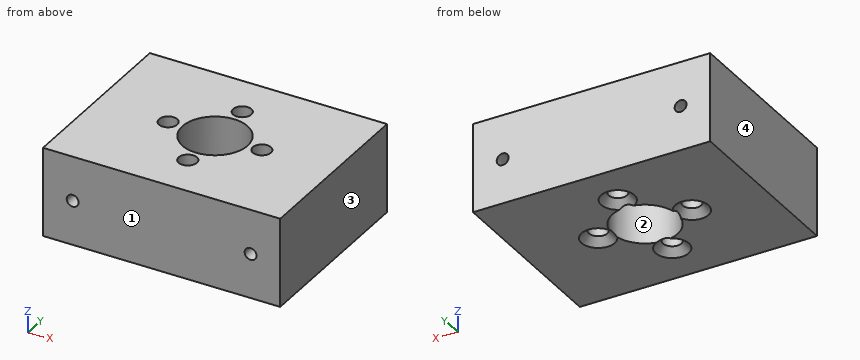
```python
from build123d import *

# Parameters (mm, degrees)
F0_W           = 40
F0_H           = 31
F1_DEPTH       = 15
F2_D           = 11
F3_D           = 3.1
F3_CSINK_D     = 5.6
F3_CSINK_ANGLE = 90
F5_D           = 2


with BuildPart() as f1:
    # F0 (on Top) → F1 (new body)
    with BuildSketch(Plane.XY):
        Rectangle(F0_W, F0_H)
    extrude(amount=F1_DEPTH)

    # F2 (through all)
    with Locations(Plane(origin=(0, 0, 0), x_dir=(1, 0, 0), z_dir=(0, 0, -1))):
        with Locations((0, 0)):
            Hole(F2_D / 2)

    # F3 (through all)
    with Locations(Plane(origin=(0, 0, 0), x_dir=(1, 0, 0), z_dir=(0, 0, -1))):
        with Locations((7.9, 0), (0, 7.9), (-7.9, 0), (0, -7.9)):
            CounterSinkHole(F3_D / 2, F3_CSINK_D / 2, counter_sink_angle=F3_CSINK_ANGLE)

    # F5 (through all)
    with Locations(Plane.XZ.offset(15.5)):
        with Locations((-15, 7.5), (15, 7.5)):
            Hole(F5_D / 2)


solid = f1.part
```
Build history of the part. All positions in model axes, mm. Face numbers are marked on the shaded views. Round coordinates to 2 decimals unless told otherwise and drop trailing zeros. Write each loop counter-clockwise with the first axis right and the second up, starting at its lowest first coordinate (ties: lowest second). Pieces come first, ordered by that corner, then holes. Notation, with made-up numbers: (21.25, 66.25) - (41.25, 66.25) arc R31 cw to (41.25, 99.25) - close; hole circle Ø2 at (56, 69). An arc over 180 degrees is marked (long way). Write each question's results on one line, items separated by ' | '. Start each with the question number.
Item 1: Saw through at B-B (y = 0). Write the cut outline in (x, z), and give its area (3 significant figures).
Item 2: Mould opens along X. For the marked faces 1, 2, 3 and 4 say: pulls with the +X half, pulls with the -X half, needs draft (parallel to the pull), parting line crosses it, or undercut.
Item 3: Saw through at D-D (z = 14). Write the cut outline in (x, y).
Item 4: Saw through at C-C (x = -7.9). Write the cut outline in (y, z).
Item 5: Drop flat-ended pins along their axis: P1, Ø4, axis at x = 7.9, y = 0, coming from the -Z side; P2, Ø3.5, axis at x = -7.9, y = 0, coming from the -Z side; P3, Ø3, axis at x = 0, y = -7.9, coming from the -Z side; P4, Ø17.5, axis at x = 0, y = 0, coming from the +Z side. Give the stop position or say it passes through.
Item 6: Saw through at A-A (z = 7.5). Write the cut outline in (x, y), and give its area (3 significant figures).
Item 7: Wall check: L1, parallel to Y at x = 0, z = 11; L2, parallel to X at y = -7.9, z = 9; L3, parallel to Y at x = -1, z = 5.75. Give the ranges that are in metal, low to high. Write a range as [from, to].
Results are:
1) outline: (-20, 0) - (-10.7, 0) - (-9.45, 1.25) - (-9.45, 15) - (-20, 15) - close; (-6.35, 1.25) - (-5.5, 0.4) - (-5.5, 15) - (-6.35, 15) - close; (5.5, 0.4) - (6.35, 1.25) - (6.35, 15) - (5.5, 15) - close; (9.45, 1.25) - (10.7, 0) - (20, 0) - (20, 15) - (9.45, 15) - close; hole circle Ø2 at (-15, 7.5); hole circle Ø2 at (15, 7.5) | area: 333 mm²
2) face 1: needs draft | face 2: undercut | face 3: pulls with the +X half | face 4: pulls with the -X half
3) outline: (-20, -15.5) - (20, -15.5) - (20, 15.5) - (-20, 15.5) - close; hole circle Ø3.1 at (-7.9, 0); hole circle Ø11 at (0, 0); hole circle Ø3.1 at (0, -7.9); hole circle Ø3.1 at (0, 7.9); hole circle Ø3.1 at (7.9, 0)
4) outline: (-15.5, 0) - (-2.8, 0) - (-1.55, 1.25) - (-1.55, 15) - (-15.5, 15) - close; (1.55, 1.25) - (2.8, 0) - (15.5, 0) - (15.5, 15) - (1.55, 15) - close
5) P1: stops at z = 0.8 | P2: stops at z = 1.05 | P3: passes through | P4: stops at z = 15
6) outline: (-20, -15.5) - (-16, -15.5) - (-16, 15.5) - (-20, 15.5) - close; (-14, -15.5) - (14, -15.5) - (14, 15.5) - (-14, 15.5) - close; (16, -15.5) - (20, -15.5) - (20, 15.5) - (16, 15.5) - close; hole circle Ø3.1 at (-7.9, 0); hole circle Ø11 at (0, 0); hole circle Ø3.1 at (0, -7.9); hole circle Ø3.1 at (0, 7.9); hole circle Ø3.1 at (7.9, 0) | area: 991 mm²
7) L1: y = [-15.5, -9.45], [-6.35, -5.5], [5.5, 6.35], [9.45, 15.5] | L2: x = [-20, -1.55], [1.55, 20] | L3: y = [-15.5, -9.08], [-6.72, -5.41], [5.41, 6.72], [9.08, 15.5]
